Verification items for the finished model (mm, model axes). A direction names the side the tool comes from. Coordinates: 2 decimals unless noted, no trailing zeros. Order: outer loops, then holes, each group sorted by start corner. A loop starts at its lowest first (then second) coordinate and runs counter-clockwise, first axis right, second up. Notation, with made-up numbers: (1, 87) - (6, 87) arc R19 cw to (6, 100) - close; hole circle Ø3 at (34, -19). An arc over 180 degrees is marked (long way). One line per question, with ' | ' between items. Start each with the question number.
from build123d import *

# Parameters (mm, degrees)
SKETCH1_W           = 191
SKETCH1_H           = 46
SKETCH1_R           = 1.549999948
BOSS_EXTRUDE1_DEPTH = 3
CUT_EXTRUDE1_REACH  = 5
SKETCH4_W           = 10
SKETCH4_H           = 3
SKETCH4_W_2         = 20
SKETCH4_W_3         = 30
CUT_EXTRUDE2_REACH  = 5
SKETCH5_W           = 3
SKETCH5_H           = 9
CUT_EXTRUDE3_REACH  = 5
SKETCH6_W           = 3
SKETCH6_H           = 9
CUT_EXTRUDE4_REACH  = 5
SKETCH7_R           = 3
CUT_EXTRUDE5_REACH  = 5
SKETCH8_R           = 1.55
CUT_EXTRUDE6_REACH  = 5
SKETCH9_R           = 1.55
CUT_EXTRUDE7_REACH  = 5
SKETCH10_R          = 1.05
CUT_EXTRUDE8_REACH  = 5
SKETCH11_R          = 1.05


with BuildPart() as part:
    # Sketch1 → Boss-Extrude1 (new body)
    with BuildSketch(Plane.XY):
        with Locations((95.5, 23)):
            Rectangle(SKETCH1_W, SKETCH1_H)
        with Locations((181, 30)):
            Circle(SKETCH1_R, mode=Mode.SUBTRACT)
        with Locations((181, 10)):
            Circle(SKETCH1_R, mode=Mode.SUBTRACT)
    extrude(amount=BOSS_EXTRUDE1_DEPTH)

    # Sketch4 → Cut-Extrude1 (cut, up to next)
    with BuildSketch(Plane(origin=(0, 0, 0), x_dir=(-1, 0, 0), z_dir=(0, 0, -1)), mode=Mode.PRIVATE) as cut_extrude1_sk1:
        with Locations((-5, 44.5)):
            Rectangle(SKETCH4_W, SKETCH4_H)
    cut_extrude1_tool1 = extrude(cut_extrude1_sk1.sketch, amount=-CUT_EXTRUDE1_REACH, mode=Mode.PRIVATE) & part.part
    add(cut_extrude1_tool1.solids().sort_by_distance((5, 44.5, 0))[0], mode=Mode.SUBTRACT)
    # Sketch4 → Cut-Extrude1 (cut, up to next)
    with BuildSketch(Plane(origin=(0, 0, 0), x_dir=(-1, 0, 0), z_dir=(0, 0, -1)), mode=Mode.PRIVATE) as cut_extrude1_sk2:
        with Locations((-25, 44.5)):
            Rectangle(SKETCH4_W, SKETCH4_H)
    cut_extrude1_tool2 = extrude(cut_extrude1_sk2.sketch, amount=-CUT_EXTRUDE1_REACH, mode=Mode.PRIVATE) & part.part
    add(cut_extrude1_tool2.solids().sort_by_distance((25, 44.5, 0))[0], mode=Mode.SUBTRACT)
    # Sketch4 → Cut-Extrude1 (cut, up to next)
    with BuildSketch(Plane(origin=(0, 0, 0), x_dir=(-1, 0, 0), z_dir=(0, 0, -1)), mode=Mode.PRIVATE) as cut_extrude1_sk3:
        with Locations((-45, 44.5)):
            Rectangle(SKETCH4_W, SKETCH4_H)
    cut_extrude1_tool3 = extrude(cut_extrude1_sk3.sketch, amount=-CUT_EXTRUDE1_REACH, mode=Mode.PRIVATE) & part.part
    add(cut_extrude1_tool3.solids().sort_by_distance((45, 44.5, 0))[0], mode=Mode.SUBTRACT)
    # Sketch4 → Cut-Extrude1 (cut, up to next)
    with BuildSketch(Plane(origin=(0, 0, 0), x_dir=(-1, 0, 0), z_dir=(0, 0, -1)), mode=Mode.PRIVATE) as cut_extrude1_sk4:
        with Locations((-70, 44.5)):
            Rectangle(SKETCH4_W_2, SKETCH4_H)
    cut_extrude1_tool4 = extrude(cut_extrude1_sk4.sketch, amount=-CUT_EXTRUDE1_REACH, mode=Mode.PRIVATE) & part.part
    add(cut_extrude1_tool4.solids().sort_by_distance((70, 44.5, 0))[0], mode=Mode.SUBTRACT)
    # Sketch4 → Cut-Extrude1 (cut, up to next)
    with BuildSketch(Plane(origin=(0, 0, 0), x_dir=(-1, 0, 0), z_dir=(0, 0, -1)), mode=Mode.PRIVATE) as cut_extrude1_sk5:
        with Locations((-116, 44.5)):
            Rectangle(SKETCH4_W_3, SKETCH4_H)
    cut_extrude1_tool5 = extrude(cut_extrude1_sk5.sketch, amount=-CUT_EXTRUDE1_REACH, mode=Mode.PRIVATE) & part.part
    add(cut_extrude1_tool5.solids().sort_by_distance((116, 44.5, 0))[0], mode=Mode.SUBTRACT)
    # Sketch4 → Cut-Extrude1 (cut, up to next)
    with BuildSketch(Plane(origin=(0, 0, 0), x_dir=(-1, 0, 0), z_dir=(0, 0, -1)), mode=Mode.PRIVATE) as cut_extrude1_sk6:
        with Locations((-146, 44.5)):
            Rectangle(SKETCH4_W, SKETCH4_H)
    cut_extrude1_tool6 = extrude(cut_extrude1_sk6.sketch, amount=-CUT_EXTRUDE1_REACH, mode=Mode.PRIVATE) & part.part
    add(cut_extrude1_tool6.solids().sort_by_distance((146, 44.5, 0))[0], mode=Mode.SUBTRACT)
    # Sketch4 → Cut-Extrude1 (cut, up to next)
    with BuildSketch(Plane(origin=(0, 0, 0), x_dir=(-1, 0, 0), z_dir=(0, 0, -1)), mode=Mode.PRIVATE) as cut_extrude1_sk7:
        with Locations((-166, 44.5)):
            Rectangle(SKETCH4_W, SKETCH4_H)
    cut_extrude1_tool7 = extrude(cut_extrude1_sk7.sketch, amount=-CUT_EXTRUDE1_REACH, mode=Mode.PRIVATE) & part.part
    add(cut_extrude1_tool7.solids().sort_by_distance((166, 44.5, 0))[0], mode=Mode.SUBTRACT)
    # Sketch4 → Cut-Extrude1 (cut, up to next)
    with BuildSketch(Plane(origin=(0, 0, 0), x_dir=(-1, 0, 0), z_dir=(0, 0, -1)), mode=Mode.PRIVATE) as cut_extrude1_sk8:
        with Locations((-186, 44.5)):
            Rectangle(SKETCH4_W, SKETCH4_H)
    cut_extrude1_tool8 = extrude(cut_extrude1_sk8.sketch, amount=-CUT_EXTRUDE1_REACH, mode=Mode.PRIVATE) & part.part
    add(cut_extrude1_tool8.solids().sort_by_distance((186, 44.5, 0))[0], mode=Mode.SUBTRACT)

    # Sketch5 → Cut-Extrude2 (cut, up to next)
    with BuildSketch(Plane(origin=(0, 0, 0), x_dir=(-1, 0, 0), z_dir=(0, 0, -1)), mode=Mode.PRIVATE) as cut_extrude2_sk1:
        with Locations((-1.5, 29.5)):
            Rectangle(SKETCH5_W, SKETCH5_H)
    cut_extrude2_tool1 = extrude(cut_extrude2_sk1.sketch, amount=-CUT_EXTRUDE2_REACH, mode=Mode.PRIVATE) & part.part
    add(cut_extrude2_tool1.solids().sort_by_distance((1.5, 29.5, 0))[0], mode=Mode.SUBTRACT)
    # Sketch5 → Cut-Extrude2 (cut, up to next)
    with BuildSketch(Plane(origin=(0, 0, 0), x_dir=(-1, 0, 0), z_dir=(0, 0, -1)), mode=Mode.PRIVATE) as cut_extrude2_sk2:
        with Locations((-1.5, 11.5)):
            Rectangle(SKETCH5_W, SKETCH5_H)
    cut_extrude2_tool2 = extrude(cut_extrude2_sk2.sketch, amount=-CUT_EXTRUDE2_REACH, mode=Mode.PRIVATE) & part.part
    add(cut_extrude2_tool2.solids().sort_by_distance((1.5, 11.5, 0))[0], mode=Mode.SUBTRACT)

    # Sketch6 → Cut-Extrude3 (cut, up to next)
    with BuildSketch(Plane(origin=(0, 0, 0), x_dir=(-1, 0, 0), z_dir=(0, 0, -1)), mode=Mode.PRIVATE) as cut_extrude3_sk1:
        with Locations((-189.5, 29.5)):
            Rectangle(SKETCH6_W, SKETCH6_H)
    cut_extrude3_tool1 = extrude(cut_extrude3_sk1.sketch, amount=-CUT_EXTRUDE3_REACH, mode=Mode.PRIVATE) & part.part
    add(cut_extrude3_tool1.solids().sort_by_distance((189.5, 29.5, 0))[0], mode=Mode.SUBTRACT)
    # Sketch6 → Cut-Extrude3 (cut, up to next)
    with BuildSketch(Plane(origin=(0, 0, 0), x_dir=(-1, 0, 0), z_dir=(0, 0, -1)), mode=Mode.PRIVATE) as cut_extrude3_sk2:
        with Locations((-189.5, 11.5)):
            Rectangle(SKETCH6_W, SKETCH6_H)
    cut_extrude3_tool2 = extrude(cut_extrude3_sk2.sketch, amount=-CUT_EXTRUDE3_REACH, mode=Mode.PRIVATE) & part.part
    add(cut_extrude3_tool2.solids().sort_by_distance((189.5, 11.5, 0))[0], mode=Mode.SUBTRACT)

    # Sketch7 → Cut-Extrude4 (cut, up to next)
    with BuildSketch(Plane.XY.offset(3), mode=Mode.PRIVATE) as cut_extrude4_sk1:
        with Locations((119.5, 23)):
            Circle(SKETCH7_R)
    cut_extrude4_tool1 = extrude(cut_extrude4_sk1.sketch, amount=-CUT_EXTRUDE4_REACH, mode=Mode.PRIVATE) & part.part
    add(cut_extrude4_tool1.solids().sort_by_distance((119.5, 23, 3))[0], mode=Mode.SUBTRACT)

    # Sketch8 → Cut-Extrude5 (cut, up to next)
    with BuildSketch(Plane.XY.offset(3), mode=Mode.PRIVATE) as cut_extrude5_sk1:
        with Locations((23.5, 13)):
            Circle(SKETCH8_R)
    cut_extrude5_tool1 = extrude(cut_extrude5_sk1.sketch, amount=-CUT_EXTRUDE5_REACH, mode=Mode.PRIVATE) & part.part
    add(cut_extrude5_tool1.solids().sort_by_distance((23.5, 13, 3))[0], mode=Mode.SUBTRACT)
    # Sketch8 → Cut-Extrude5 (cut, up to next)
    with BuildSketch(Plane.XY.offset(3), mode=Mode.PRIVATE) as cut_extrude5_sk2:
        with Locations((23.5, 23)):
            Circle(SKETCH8_R)
    cut_extrude5_tool2 = extrude(cut_extrude5_sk2.sketch, amount=-CUT_EXTRUDE5_REACH, mode=Mode.PRIVATE) & part.part
    add(cut_extrude5_tool2.solids().sort_by_distance((23.5, 23, 3))[0], mode=Mode.SUBTRACT)
    # Sketch8 → Cut-Extrude5 (cut, up to next)
    with BuildSketch(Plane.XY.offset(3), mode=Mode.PRIVATE) as cut_extrude5_sk3:
        with Locations((53.5, 32)):
            Circle(SKETCH8_R)
    cut_extrude5_tool3 = extrude(cut_extrude5_sk3.sketch, amount=-CUT_EXTRUDE5_REACH, mode=Mode.PRIVATE) & part.part
    add(cut_extrude5_tool3.solids().sort_by_distance((53.5, 32, 3))[0], mode=Mode.SUBTRACT)
    # Sketch8 → Cut-Extrude5 (cut, up to next)
    with BuildSketch(Plane.XY.offset(3), mode=Mode.PRIVATE) as cut_extrude5_sk4:
        with Locations((68.757359313, 10.5)):
            Circle(SKETCH8_R)
    cut_extrude5_tool4 = extrude(cut_extrude5_sk4.sketch, amount=-CUT_EXTRUDE5_REACH, mode=Mode.PRIVATE) & part.part
    add(cut_extrude5_tool4.solids().sort_by_distance((68.757359, 10.5, 3))[0], mode=Mode.SUBTRACT)
    # Sketch8 → Cut-Extrude5 (cut, up to next)
    with BuildSketch(Plane.XY.offset(3), mode=Mode.PRIVATE) as cut_extrude5_sk5:
        with Locations((80.757359313, 10.5)):
            Circle(SKETCH8_R)
    cut_extrude5_tool5 = extrude(cut_extrude5_sk5.sketch, amount=-CUT_EXTRUDE5_REACH, mode=Mode.PRIVATE) & part.part
    add(cut_extrude5_tool5.solids().sort_by_distance((80.757359, 10.5, 3))[0], mode=Mode.SUBTRACT)

    # Sketch9 → Cut-Extrude6 (cut, up to next)
    with BuildSketch(Plane(origin=(0, 0, 0), x_dir=(-1, 0, 0), z_dir=(0, 0, -1)), mode=Mode.PRIVATE) as cut_extrude6_sk1:
        with Locations((-137.2, 7.8)):
            Circle(SKETCH9_R)
    cut_extrude6_tool1 = extrude(cut_extrude6_sk1.sketch, amount=-CUT_EXTRUDE6_REACH, mode=Mode.PRIVATE) & part.part
    add(cut_extrude6_tool1.solids().sort_by_distance((137.2, 7.8, 0))[0], mode=Mode.SUBTRACT)
    # Sketch9 → Cut-Extrude6 (cut, up to next)
    with BuildSketch(Plane(origin=(0, 0, 0), x_dir=(-1, 0, 0), z_dir=(0, 0, -1)), mode=Mode.PRIVATE) as cut_extrude6_sk2:
        with Locations((-6.5, 7.8)):
            Circle(SKETCH9_R)
    cut_extrude6_tool2 = extrude(cut_extrude6_sk2.sketch, amount=-CUT_EXTRUDE6_REACH, mode=Mode.PRIVATE) & part.part
    add(cut_extrude6_tool2.solids().sort_by_distance((6.5, 7.8, 0))[0], mode=Mode.SUBTRACT)

    # Sketch10 → Cut-Extrude7 (cut, up to next)
    with BuildSketch(Plane.XY.offset(3), mode=Mode.PRIVATE) as cut_extrude7_sk1:
        with Locations((93, 25)):
            Circle(SKETCH10_R)
    cut_extrude7_tool1 = extrude(cut_extrude7_sk1.sketch, amount=-CUT_EXTRUDE7_REACH, mode=Mode.PRIVATE) & part.part
    add(cut_extrude7_tool1.solids().sort_by_distance((93, 25, 3))[0], mode=Mode.SUBTRACT)
    # Sketch10 → Cut-Extrude7 (cut, up to next)
    with BuildSketch(Plane.XY.offset(3), mode=Mode.PRIVATE) as cut_extrude7_sk2:
        Polygon((83, 24), (83, 34), (82, 35), (75, 35), (74, 34), (74, 24), (75, 23), (82, 23), align=None)
    cut_extrude7_tool2 = extrude(cut_extrude7_sk2.sketch, amount=-CUT_EXTRUDE7_REACH, mode=Mode.PRIVATE) & part.part
    add(cut_extrude7_tool2.solids().sort_by_distance((78.5, 29, 3))[0], mode=Mode.SUBTRACT)

    # Sketch11 → Cut-Extrude8 (cut, up to next)
    with BuildSketch(Plane.XY.offset(3), mode=Mode.PRIVATE) as cut_extrude8_sk1:
        Polygon((164, 23), (157, 23), (156, 24), (156, 34), (157, 35), (164, 35), (165, 34), (165, 24), align=None)
    cut_extrude8_tool1 = extrude(cut_extrude8_sk1.sketch, amount=-CUT_EXTRUDE8_REACH, mode=Mode.PRIVATE) & part.part
    add(cut_extrude8_tool1.solids().sort_by_distance((160.5, 29, 3))[0], mode=Mode.SUBTRACT)
    # Sketch11 → Cut-Extrude8 (cut, up to next)
    with BuildSketch(Plane.XY.offset(3), mode=Mode.PRIVATE) as cut_extrude8_sk2:
        with Locations((146, 25)):
            Circle(SKETCH11_R)
    cut_extrude8_tool2 = extrude(cut_extrude8_sk2.sketch, amount=-CUT_EXTRUDE8_REACH, mode=Mode.PRIVATE) & part.part
    add(cut_extrude8_tool2.solids().sort_by_distance((146, 25, 3))[0], mode=Mode.SUBTRACT)


solid = part.part
Item 1: Section check A-A (z = 2.45). Give the number of separate pieces and of enclosed holes in the cut face, then the cut area to 3 significant figures.
Item 2: Set-up check for faces 5 (the flat face through (3, 29, 1)), 6 (the flat face through (83, 29, 2)), 7 (the flat face through (186, 43, 1)): record each of +Z, -Z, +X, -X, +Y, -Y from which the full face is reachable in a straight line by a thin tool's end or side.
Item 3: Mould release check, pull along Y, two halves, no side actions. Record for faces 1 (the flat face through (101, 44, 1)), 2 (the flat face through (190, 25, 1)), 3 (the cylindrical face through (23.298, 24.537, 1.521)), 4 (the flat face through (90, 46, 1)): +Y half, -Y half, draft (parallel to the pull), parting line (faces both ways), or undercut.
Item 4: Thickness scan on probe 1 along Y at (x, z) = (137.2, 1.15); probe 2 along X at (y, z) = (29, 1.5); probe 3 along Y at (x, z) = (53.5, 1.1). Record the ranges inside material, lowest first. Write a range as from..to.
Item 5: Section check B-B (x = 127.5). Record the cut outline in (y, z).
Item 6: Gauge pin test, flat ends, axial feed: pin 1 (1.5 mm diameter, centred on x = 189, z = 1.5, fed in from +Y); pin 2 (1.5 mm diameter, centred on y = 27.5, z = 2, fed in from -X); pin 3 (1.5 mm diameter, centred on y = 45, z = 2, fed in from +X). Record the tip position at first contact, or that the pin passes through.
Completed:
1) separate pieces: 1 | enclosed holes: 14 | area: 8,030 mm^2
2) face 5: +Z, -Z, -X | face 6: +Z, -Z | face 7: +Z, -Z, +X, +Y
3) face 1: draft | face 2: undercut | face 3: undercut | face 4: +Y half
4) probe 1: y = 0..6.25, 9.35..46 | probe 2: x = 3..74, 83..156, 165..179.82, 182.18..188 | probe 3: y = 0..30.45, 33.55..46
5) outline: (0, 0) - (43, 0) - (43, 3) - (0, 3) - close
6) pin 1: stops at y = 43 | pin 2: stops at x = 3 | pin 3: stops at x = 181
